For this review, take the finished solid that the model builds, in its own axes (mm). Face numbers are marked on the shaded views. A direction names the side the tool comes from. Coordinates: 2 decimals unless noted, no trailing zeros. Write each loop counter-clockwise with the first axis right and the second up, starting at its lowest first coordinate (ties: lowest second). Pieces come first, ordered by that corner, then holes.
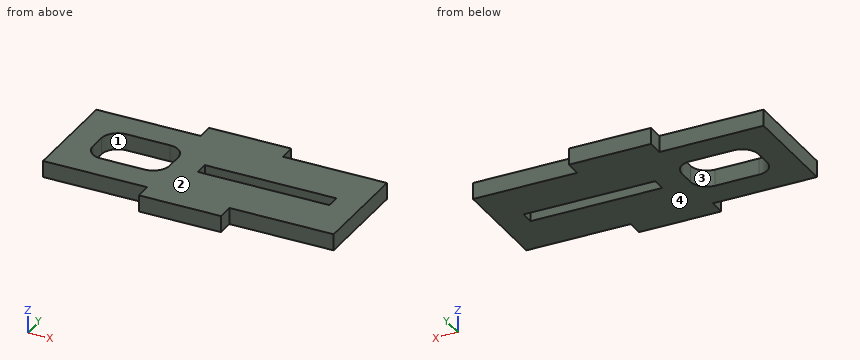
```python
from build123d import *

# Parameters (mm, degrees)
SKETCH1_W           = 24
SKETCH1_H           = 2.5
BOSS_EXTRUDE1_DEPTH = 3


with BuildPart() as part:
    # Sketch1 → Boss-Extrude1 (new body)
    with BuildSketch(Plane.XY):
        Polygon((-26.5, -9.5), (-26.5, 9.5), (-7.5, 9.5), (-7.5, 12.5), (7.5, 12.5), (7.5, 9.5), (26.5, 9.5), (26.5, -9.5), (7.5, -9.5), (7.5, -12.5), (-7.5, -12.5), (-7.5, -9.5), align=None)
        with Locations((9.5, 0)):
            Rectangle(SKETCH1_W, SKETCH1_H, mode=Mode.SUBTRACT)
        with BuildLine():
            Line((-18.5, 4.5), (-10.5, 4.5))
            ThreePointArc((-10.5, 4.5), (-8.378679656, 3.621320344), (-7.5, 1.5))
            Line((-7.5, 1.5), (-7.5, -1.5))
            ThreePointArc((-7.5, -1.5), (-8.378679656, -3.621320344), (-10.5, -4.5))
            Line((-10.5, -4.5), (-18.5, -4.5))
            ThreePointArc((-18.5, -4.5), (-20.621320344, -3.621320344), (-21.5, -1.5))
            Line((-21.5, -1.5), (-21.5, 1.5))
            ThreePointArc((-21.5, 1.5), (-20.621320344, 3.621320344), (-18.5, 4.5))
        make_face(mode=Mode.SUBTRACT)
    extrude(amount=BOSS_EXTRUDE1_DEPTH)


solid = part.part
```
1) Consider section B-B (x = -2). Give the boundary of the cut face in (y, z).
2) Clearance check with flat-ended pins moving along their axes: P1, Ø1.5, axis at y = 10.5, z = 2, coming from the -X side; P2, Ø0.9, axis at x = -18, z = 1.5, coming from the +Y side. State where each tip first meets the part, or that it passes through.
3) The part is to be moulded in two halves that separate along Y. For the marked faces 3 and 4, say which applies: pulls with the +Y half, pulls with the -Y half, needs draft (parallel to the pull), parting line crosses it, or undercut.
4) Tool access review of the marked faces 1 and 2: name each direction out of +Z, -Z, +X, -X, +Y, -Y from which nothing blocks a thin tool from reaching the whole face with its end or side.
5) Consider section D-D (y = -3.5). Give the boundary of the cut face in (x, z).
6) For L1, parallel to Y at x = 11, z = 0.55; L2, parallel to Y at x = -14.5, z = 0.2; L3, parallel to X at y = 10.5, z = 2, list the stretches that pass through material, from the lowest coordinate up.
7) Consider section C-C (z = 0.8). Give the boundary of the cut face in (x, y).
8) Consider section A-A (y = 0.5). Give the boundary of the cut face in (x, z).
Results:
1. outline: (-12.5, 0) - (-1.25, 0) - (-1.25, 3) - (-12.5, 3) - close; (1.25, 0) - (12.5, 0) - (12.5, 3) - (1.25, 3) - close
2. P1: stops at x = -7.5
2. P2: stops at y = 9.5
3. face 3: undercut
3. face 4: needs draft
4. face 1: +Z, -Z
4. face 2: +Z, +X, -X, +Y, -Y
5. outline: (-26.5, 0) - (-20.74, 0) - (-20.74, 3) - (-26.5, 3) - close; (-8.26, 0) - (26.5, 0) - (26.5, 3) - (-8.26, 3) - close
6. L1: y = -9.5 to -1.25, 1.25 to 9.5
6. L2: y = -9.5 to -4.5, 4.5 to 9.5
6. L3: x = -7.5 to 7.5
7. outline: (-26.5, -9.5) - (-7.5, -9.5) - (-7.5, -12.5) - (7.5, -12.5) - (7.5, -9.5) - (26.5, -9.5) - (26.5, 9.5) - (7.5, 9.5) - (7.5, 12.5) - (-7.5, 12.5) - (-7.5, 9.5) - (-26.5, 9.5) - close; hole (-21.5, -1.5) arc R3 ccw to (-18.5, -4.5) - (-10.5, -4.5) arc R3 ccw to (-7.5, -1.5) - (-7.5, 1.5) arc R3 ccw to (-10.5, 4.5) - (-18.5, 4.5) arc R3 ccw to (-21.5, 1.5) - close; hole (-2.5, -1.25) - (21.5, -1.25) - (21.5, 1.25) - (-2.5, 1.25) - close
8. outline: (-26.5, 0) - (-21.5, 0) - (-21.5, 3) - (-26.5, 3) - close; (-7.5, 0) - (-2.5, 0) - (-2.5, 3) - (-7.5, 3) - close; (21.5, 0) - (26.5, 0) - (26.5, 3) - (21.5, 3) - close
